Part model, mm, in its own coordinate system. A direction names the side the tool comes from. Coordinates: 2 decimals unless noted, no trailing zeros. Order: outer loops, then holes, each group sorted by start corner. A loop starts at its lowest first (then second) coordinate and runs counter-clockwise, first axis right, second up. Notation, with made-up numbers: (43.5, -11.75) - (62.5, -11.75) arc R8 cw to (62.5, -6.75) - close; hole circle Ø7 at (-37, 46.5). An arc over 180 degrees is marked (long way). Use a Markdown table: item, result. Add a question column.
1) Wall check: L1, parallel to Y at x = 29.6, z = 0; L2, parallel to Z at x = 30.5, y = 11.5; L3, parallel to Y at x = 28, z = 11. Give the ranges that are in metal, low to high. Write a range as [from, to].
2) Tool access for faces 4 (the face through (11.6, -7, -2)), 5 (the face through (4.2, -9, 4)), 6 (the face through (3, -9, -4)): list every direction of +Z, -Z, +X, -X, +Y, -Y with a clear straight run to the whole face (end or side of a thin tool).
3) Two-plate mould, pull along Y, no slides. Class faces 1 (the face through (21, 0, 16)), 2 (the face through (21.01, 15.1, 15.14)), 3 (the face through (29.365, 23.417, -0.759)): +Y half, -Y half, draft (parallel to the pull), parting line (faces both ways), or undercut.
4) Saw through at A-A on x = 9. List the corners of the cut face in (y, z), then the cut area to 3 significant figures.
5) Saw through at D-D on z = 0. Count the separate pieces of the cut face and the enclosed holes in it, then the cut area to 3 significant figures.
6) Drop flat-ended pins along their axis: P1, Ø5, axis at x = 23.5, z = 1, coming from the +Y side; P2, Ø18.5, axis at y = -1.5, z = 0.5, coming from the +X side; P3, Ø1.5, axis at x = 4.5, y = 13, coming from the -Z side; P4, Ø2, axis at y = 11.5, z = -11.5, coming from the +X side. Give the stop position or say it passes through.
7) Saw through at B-B on y = 0. List the corners of the cut face in (x, z).
```python
from build123d import *

# Parameters (mm, degrees)
SKETCH_2_R               = 9
EXTRUDE_1_DEPTH          = 25
SKETCH_3_R               = 11
EXTRUDE_2_DEPTH          = 12
SKETCH_4_R               = 9
EXTRUDE_3_DEPTH          = 6
SKETCH_5_R               = 10.75
CUT_EXTRUDE_1_DEPTH      = 23.1
CUT_EXTRUDE_START        = -8.5
SKETCH_6_R               = 8.5
CUT_EXTRUDE_2_DEPTH      = 7
CUT_EXTRUDE_3_REACH      = 59.899
CUT_EXTRUDE_3_END_RADIUS = 10.75
SKETCH_8_R               = 6.75
SKETCH_9_R               = 3.5
CUT_EXTRUDE_4_DEPTH      = 58.524690439
SKETCH_10_R              = 10.75
EXTRUDE_4_DEPTH          = 5.95
CHAMFER_1_SIZE           = 0.828
SKETCH_12_W              = 32
SKETCH_12_H              = 32
SKETCH_12_R              = 15
EXTRUDE_5_DEPTH          = 27
CUT_EXTRUDE_5_REACH      = 51.841
SKETCH_13_R              = 6.75
CUT_EXTRUDE_6_REACH      = 72.293
SKETCH_14_R              = 7.172
CUT_EXTRUDE_11_REACH     = 56.144
SKETCH_18_R              = 10.75
M3X0_51_D                = 2.5
M3X0_51_DEPTH            = 8.5
M3X0_51_CSINK_D          = 3.05
M3X0_51_CSINK_ANGLE      = 90
M3X0_51_TIP              = 0.751075774
FILLET_1_R               = 3
CHAMFER_2_SIZE           = 1


with BuildPart() as part:
    # Эскиз1 → Повернуть1 (revolve)
    with BuildSketch(Plane.XY, mode=Mode.PRIVATE) as revolve_1_sk:
        Polygon((0, -7), (11.6, -7), (11.6, 0), (34.7, 0), (34.7, -10.5), (34.7, -16), (7.7, -16), (7.7, -9.5), (4.2, -9.5), (4.2, -11.5), (3, -11.5), (3, -9.5), (0, -9.5), align=None)
    revolve(revolve_1_sk.sketch.rotate(Axis((0, 0, 0), (1, 0, 0)), 270), axis=Axis((0, 0, 0), (1, 0, 0)))

    # Эскиз2 → Бобышка-Вытянуть1 (add)
    with BuildSketch(Plane(origin=(0, 0, 0), x_dir=(1, 0, 0), z_dir=(0, 1, 0))):
        with Locations(Location((22, 0, 0), (0, 0, 90))):
            Circle(SKETCH_2_R)
    extrude(amount=EXTRUDE_1_DEPTH)

    # Эскиз3 → Бобышка-Вытянуть2 (add)
    with BuildSketch(Plane(origin=(0, 25, 0), x_dir=(1, 0, 0), z_dir=(0, 1, 0))):
        with Locations(Location((22, 0, 0), (0, 0, 270))):
            Circle(SKETCH_3_R)
    extrude(amount=EXTRUDE_2_DEPTH)

    # Эскиз4 → Бобышка-Вытянуть3 (add)
    with BuildSketch(Plane(origin=(0, 37, 0), x_dir=(1, 0, 0), z_dir=(0, 1, 0))):
        with Locations(Location((22, 0, 0), (0, 0, 90))):
            Circle(SKETCH_4_R)
    extrude(amount=EXTRUDE_3_DEPTH)

    # Эскиз5 → Вырез-Вытянуть1 (cut)
    with BuildSketch(Plane(origin=(34.7, 0, 0), x_dir=(0, 0, -1), z_dir=(1, 0, 0))):
        Circle(SKETCH_5_R)
    extrude(amount=-CUT_EXTRUDE_1_DEPTH, mode=Mode.SUBTRACT)

    # Эскиз6 → Вырез-Вытянуть2 (cut)
    with BuildSketch(Plane(origin=(0, 43, 0), x_dir=(1, 0, 0), z_dir=(0, 1, 0)).offset(CUT_EXTRUDE_START)):
        with Locations(Location((22, 0, 0), (0, 0, 270))):
            Circle(SKETCH_6_R)
    extrude(amount=-CUT_EXTRUDE_2_DEPTH, mode=Mode.SUBTRACT)

    # Вырез-Вытянуть3: up to this cylinder (the profile starts outside it)
    cut_extrude_3_end = Plane(origin=(22, 0, 0), z_dir=(1, 0, 0)) * Cylinder(CUT_EXTRUDE_3_END_RADIUS, 142.298, mode=Mode.PRIVATE)
    # Эскиз8 → Вырез-Вытянуть3 (cut, up to the surface)
    with BuildSketch(Plane(origin=(0, 27.5, 0), x_dir=(1, 0, 0), z_dir=(0, 1, 0)), mode=Mode.PRIVATE) as cut_extrude_3_sk1:
        with Locations(Location((22, 0, 0), (0, 0, 270))):
            Circle(SKETCH_8_R)
    cut_extrude_3_tool1 = extrude(cut_extrude_3_sk1.sketch, amount=-CUT_EXTRUDE_3_REACH, mode=Mode.PRIVATE) - cut_extrude_3_end
    add(cut_extrude_3_tool1.solids().sort_by_distance((22, 27.5, 0))[0], mode=Mode.SUBTRACT)

    # Эскиз9 → Вырез-Вытянуть4 (cut, through all)
    with BuildSketch(Plane(origin=(0, 0, 0), x_dir=(0, 0, -1), z_dir=(1, 0, 0))):
        with Locations(Location((0, 20, 0), (0, 0, 180))):
            Circle(SKETCH_9_R)
    extrude(amount=CUT_EXTRUDE_4_DEPTH, mode=Mode.SUBTRACT)

    # Эскиз10 → Бобышка-Вытянуть4 (add)
    with BuildSketch(Plane(origin=(34.7, 0, 0), x_dir=(0, 0, -1), z_dir=(1, 0, 0))):
        with Locations(Location((0, 0, 0), (0, 0, 90))):
            Circle(SKETCH_10_R)
    extrude(amount=-EXTRUDE_4_DEPTH)

    # Фаска1
    chamfer_1_edges = [part.edges().sort_by_distance(p)[0] for p in [
        (22, 37, -11),
    ]]
    chamfer(chamfer_1_edges, length=CHAMFER_1_SIZE)

    # Эскиз12 → Бобышка-Вытянуть5 (add)
    with BuildSketch(Plane(origin=(34.7, 0, 0), x_dir=(0, 0, -1), z_dir=(1, 0, 0))):
        Rectangle(SKETCH_12_W, SKETCH_12_H)
        Circle(SKETCH_12_R, mode=Mode.SUBTRACT)
    extrude(amount=-EXTRUDE_5_DEPTH)

    # Эскиз13 → Вырез-Вытянуть5 (cut, up to next)
    with BuildSketch(Plane(origin=(0, 16, 0), x_dir=(1, 0, 0), z_dir=(0, 1, 0)), mode=Mode.PRIVATE) as cut_extrude_5_sk1:
        with Locations(Location((22, 0, 0), (0, 0, 270))):
            Circle(SKETCH_13_R)
    cut_extrude_5_tool1 = extrude(cut_extrude_5_sk1.sketch, amount=-CUT_EXTRUDE_5_REACH, mode=Mode.PRIVATE) & part.part
    add(cut_extrude_5_tool1.solids().sort_by_distance((22, 16, 0))[0], mode=Mode.SUBTRACT)

    # Эскиз14 → Вырез-Вытянуть6 (cut, up to next)
    with BuildSketch(Plane(origin=(0, 43, 0), x_dir=(1, 0, 0), z_dir=(0, 1, 0)), mode=Mode.PRIVATE) as cut_extrude_6_sk1:
        with Locations(Location((22, 0, 0), (0, 0, 270))):
            Circle(SKETCH_14_R)
    cut_extrude_6_tool1 = extrude(cut_extrude_6_sk1.sketch, amount=-CUT_EXTRUDE_6_REACH, mode=Mode.PRIVATE) & part.part
    add(cut_extrude_6_tool1.solids().sort_by_distance((22, 43, 0))[0], mode=Mode.SUBTRACT)

    # Эскиз18 → Вырез-Вытянуть11 (cut, up to next)
    with BuildSketch(Plane.ZY.offset(-28.75), mode=Mode.PRIVATE) as cut_extrude_11_sk1:
        with Locations(Location((0, 0, 0), (0, 0, 180))):
            Circle(SKETCH_18_R)
    cut_extrude_11_tool1 = extrude(cut_extrude_11_sk1.sketch, amount=-CUT_EXTRUDE_11_REACH, mode=Mode.PRIVATE) & part.part
    add(cut_extrude_11_tool1.solids().sort_by_distance((28.75, 0, 0))[0], mode=Mode.SUBTRACT)

    # Отверстие обработанное метчиком M3x0.51
    with Locations(Plane(origin=(34.7, 11.5, 11.5), x_dir=(0, 0, 1), z_dir=(1, 0, 0))):
        with Locations((0, 0), (0, 23), (-23, 23), (-23, 0)):
            CounterSinkHole(M3X0_51_D / 2, M3X0_51_CSINK_D / 2, depth=M3X0_51_DEPTH, counter_sink_angle=M3X0_51_CSINK_ANGLE)
            with Locations((0, 0, -(M3X0_51_DEPTH + M3X0_51_TIP / 2))):  # 118° drill point
                Cone(0, M3X0_51_D / 2, M3X0_51_TIP, mode=Mode.SUBTRACT)

    # Скругление1
    fillet_1_edges = [part.edges().sort_by_distance(p)[0] for p in [
        (21.2, 16, -16),
        (21.2, -16, -16),
        (21.2, -16, 16),
        (21.2, 16, 16),
    ]]
    fillet(fillet_1_edges, radius=FILLET_1_R)

    # Фаска2
    chamfer_2_edges = [part.edges().sort_by_distance(p)[0] for p in [
        (34.7, 0, 10.75),
    ]]
    chamfer(chamfer_2_edges, length=CHAMFER_2_SIZE)


solid = part.part
```
Results are:
| question | item | result |
|---|---|---|
| 1 | L1 | [-16, -10.75], [10.75, 16.5], [23.5, 27.5], [34.5, 43] |
| 1 | L2 | [-16, -12.75], [-10.25, 10.25], [12.75, 16] |
| 1 | L3 | [-16, -12.65], [-10.35, 10.35], [12.65, 16] |
| 2 | face 4 | +X |
| 2 | face 5 | none |
| 2 | face 6 | -X |
| 3 | face 1 | draft |
| 3 | face 2 | +Y half |
| 3 | face 3 | undercut |
| 4 | outline | (-16, -13) arc R3 ccw to (-13, -16) - (13, -16) arc R3 ccw to (16, -13) - (16, 13) arc R3 ccw to (13, 16) - (-13, 16) arc R3 ccw to (-16, 13) - close; hole circle Ø14 at (0, 0) |
| 4 | area | 862 mm2 |
| 5 | separate pieces | 5 |
| 5 | enclosed holes | 0 |
| 5 | area | 390 mm2 |
| 6 | P1 | y = -10.16 |
| 6 | P2 | x = 33.78 |
| 6 | P3 | through |
| 6 | P4 | x = 26.05 |
| 7 | outline | (0, -9.5) - (3, -9.5) - (3, -11.5) - (4.2, -11.5) - (4.2, -9.5) - (7.7, -9.5) - (7.7, -16) - (34.7, -16) - (34.7, -11.75) - (33.7, -10.75) - (11.6, -10.75) - (11.6, -7) - (0, -7) - close; (0, 7) - (11.6, 7) - (11.6, 10.75) - (33.7, 10.75) - (34.7, 11.75) - (34.7, 16) - (7.7, 16) - (7.7, 9.5) - (4.2, 9.5) - (4.2, 11.5) - (3, 11.5) - (3, 9.5) - (0, 9.5) - close |
